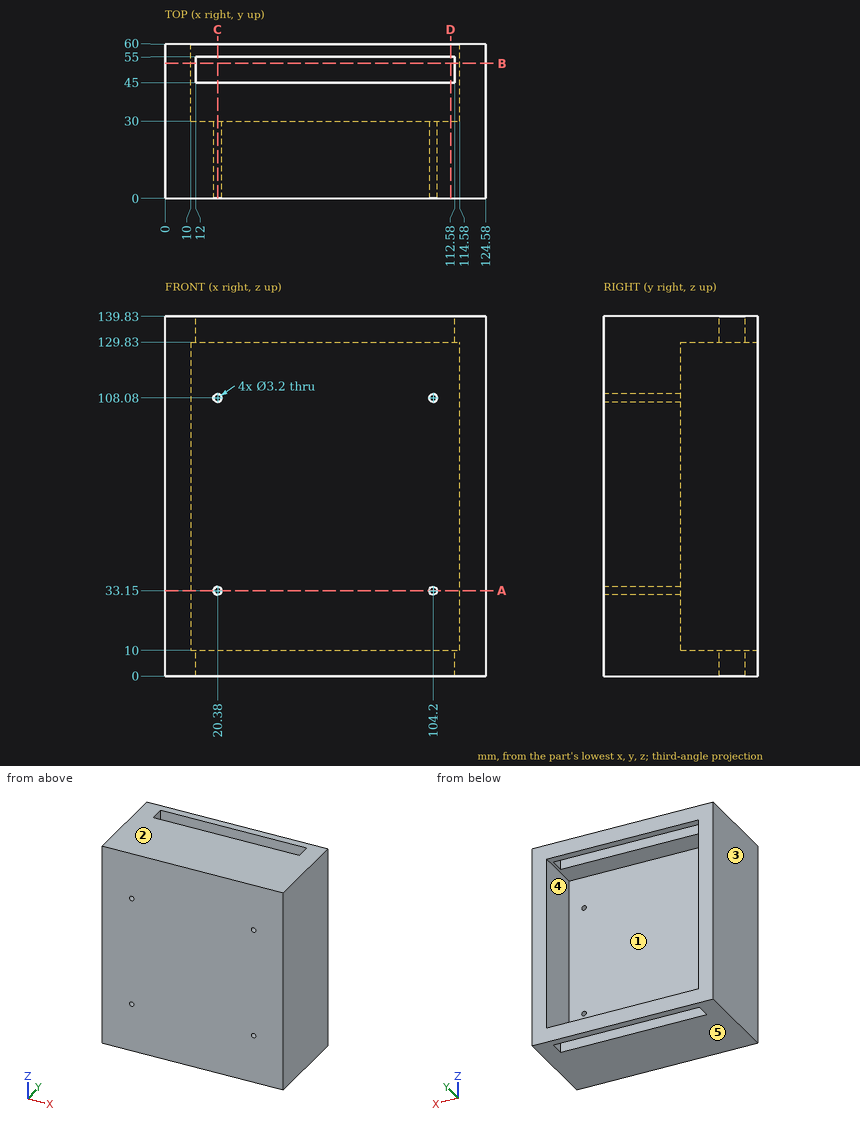
Could you check a few things on this drawing? It's one solid part, dimensions in mm from its lowest x, y, z. A direction names the side the tool comes from. Give positions to 0.01 mm unless a question says otherwise; leave off trailing zeros. Order: outer loops, then holes, each group sorted by start corner. A loop starts at its lowest first (then second) coordinate and runs counter-clockwise, first axis right, second up.
1. Which directions (+Z, -Z, +X, -X, +Y, -Y) give clear straight access to the entire face, cutting with the end or side of a thin tool? Please do the marked faces 4 and 5.
Answers below:
face 4: +Y
face 5: -Z, +X, -X, +Y, -Y
2. Suppose I cut it at C-C (x = 20.38). Write out the boundary of the cut face in (y, z), plus the area to 3 significant figures.
Answers below:
outline: (0, 0) - (45, 0) - (45, 10) - (30, 10) - (30, 31.55) - (0, 31.55) - close; (0, 34.75) - (30, 34.75) - (30, 106.48) - (0, 106.48) - close; (0, 109.68) - (30, 109.68) - (30, 129.83) - (45, 129.83) - (45, 139.83) - (0, 139.83) - close; (55, 0) - (60, 0) - (60, 10) - (55, 10) - close; (55, 129.83) - (60, 129.83) - (60, 139.83) - (55, 139.83) - close
area: 4,400 mm2
3. Suppose I cut it at A-A (z = 33.15). Write out the boundary of the cut face in (x, y), plus the area to 3 significant figures.
Answers below:
outline: (0, 0) - (18.78, 0) - (18.78, 30) - (10, 30) - (10, 60) - (0, 60) - close; (21.98, 0) - (102.6, 0) - (102.6, 30) - (21.98, 30) - close; (105.8, 0) - (124.58, 0) - (124.58, 60) - (114.58, 60) - (114.58, 30) - (105.8, 30) - close
area: 4,150 mm2
4. Suppose I cut it at D-D (x = 111). Write out the boundary of the cut face in (y, z).
Answers below:
outline: (0, 0) - (45, 0) - (45, 10) - (30, 10) - (30, 129.83) - (45, 129.83) - (45, 139.83) - (0, 139.83) - close; (55, 0) - (60, 0) - (60, 10) - (55, 10) - close; (55, 129.83) - (60, 129.83) - (60, 139.83) - (55, 139.83) - close
5. Thinking about a two-plate mould opening in X: for the marked faces 1, 2 and 3, which applies, +X half, -X half, draft (parallel to the pull), parting line (faces both ways), or undercut?
Answers below:
face 1: undercut
face 2: draft
face 3: -X half
6. I need wall thicknesses on L1, parallel to X at y = 10, z = 33; L2, parallel to Z at x = 20.38, y = 8.75; L3, parallel to Z at x = 52.5, y = 37. Which ranges of each line are inside material? Lowest first, please.
Answers below:
L1: x = 0 to 18.79, 21.97 to 102.61, 105.79 to 124.58
L2: z = 0 to 31.55, 34.75 to 106.48, 109.68 to 139.83
L3: z = 0 to 10, 129.83 to 139.83
7. Suppose I cut it at B-B (y = 52.5). Write out the boundary of the cut face in (x, z), plus the area to 3 significant figures.
Answers below:
outline: (0, 0) - (12, 0) - (12, 10) - (10, 10) - (10, 129.83) - (12, 129.83) - (12, 139.83) - (0, 139.83) - close; (112.58, 0) - (124.58, 0) - (124.58, 139.83) - (112.58, 139.83) - (112.58, 129.83) - (114.58, 129.83) - (114.58, 10) - (112.58, 10) - close
area: 2,880 mm2
8. For pin 1 (8 mm diameter, centred on x = 68.5, z = 132.5, fed in from -Y); pin 2 (2 mm diameter, centred on x = 78, z = 106, fed in from +Y), each with a flat end and sliding along its axis, tell me the tip position at first contact or that it passes through.
Answers below:
pin 1: stops at y = 0
pin 2: stops at y = 30
